Geometry check sheet. Reference: the model listing, model coordinates, mm. Face numbers are marked on the shaded views. Give positions to 0.01 mm unless a question says otherwise; leave off trailing zeros. Loops run counter-clockwise (first coordinate to the right, second up) from the corner with the lowest first, then second, coordinate; pieces in that order, holes last.
1. Release check for a two-part mould opening along Y. For the marked faces 1, 2 and 3 record: +Y half, -Y half, draft (parallel to the pull), parting line (faces both ways), or undercut.
2. Cross-section at C-C, the plane x = 1. Record the cut outline in (y, z), plus the area to 3 significant figures.
3. Go/stop test with flat-tipped pins: pin 1 Ø10 at (y, z) = (-5, 7) entering from +X; pin 2 Ø3 at (x, z) = (1, -5) entering from +Y; pin 3 Ø3 at (x, y) = (-1.5, 5) entering from +Z; pin 4 Ø1 at (x, z) = (2, 3.5) entering from +Y. Record where each tip stops, or that it passes through.
4. Material ranges on L1, parallel to Y at x = 0.5, z = 0; L2, parallel to X at y = -5.5, z = -0.25; L3, parallel to Y at x = 0.5, z = 0.75, recorded low to high.
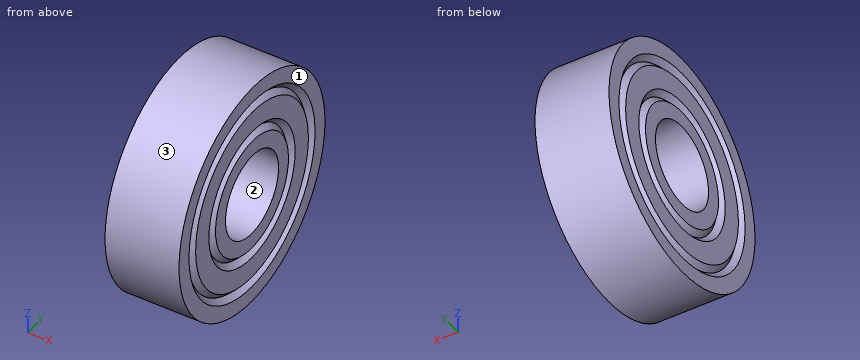
from build123d import *


with BuildPart() as part:
    # Esquisse1 → Base-Révolution (revolve)
    with BuildSketch(Plane.XY, mode=Mode.PRIVATE) as base_r_volution_sk:
        Polygon((-3.5, 4), (3.5, 4), (3.5, 5.5), (3, 6), (3.5, 6.5), (3.5, 8.5), (3, 9), (3.5, 9.5), (3.5, 11), (-3.5, 11), (-3.5, 9.5), (-3, 9), (-3.5, 8.5), (-3.5, 6.5), (-3, 6), (-3.5, 5.5), align=None)
    revolve(base_r_volution_sk.sketch.rotate(Axis((0, 0, 0), (1, 0, 0)), 90), axis=Axis((0, 0, 0), (1, 0, 0)))


solid = part.part
Result:
1. face 1: draft
1. face 2: undercut
1. face 3: parting line
2. outline: circle Ø22 at (0, 0); hole circle Ø8 at (0, 0)
2. area: 330 mm2
3. pin 1: stops at x = 3.5
3. pin 2: stops at y = 10.43
3. pin 3: stops at z = 10.43
3. pin 4: stops at y = 10.58
4. L1: y = -11 to -4, 4 to 11
4. L2: x = -3.49 to 3.49
4. L3: y = -10.97 to -3.93, 3.93 to 10.97
